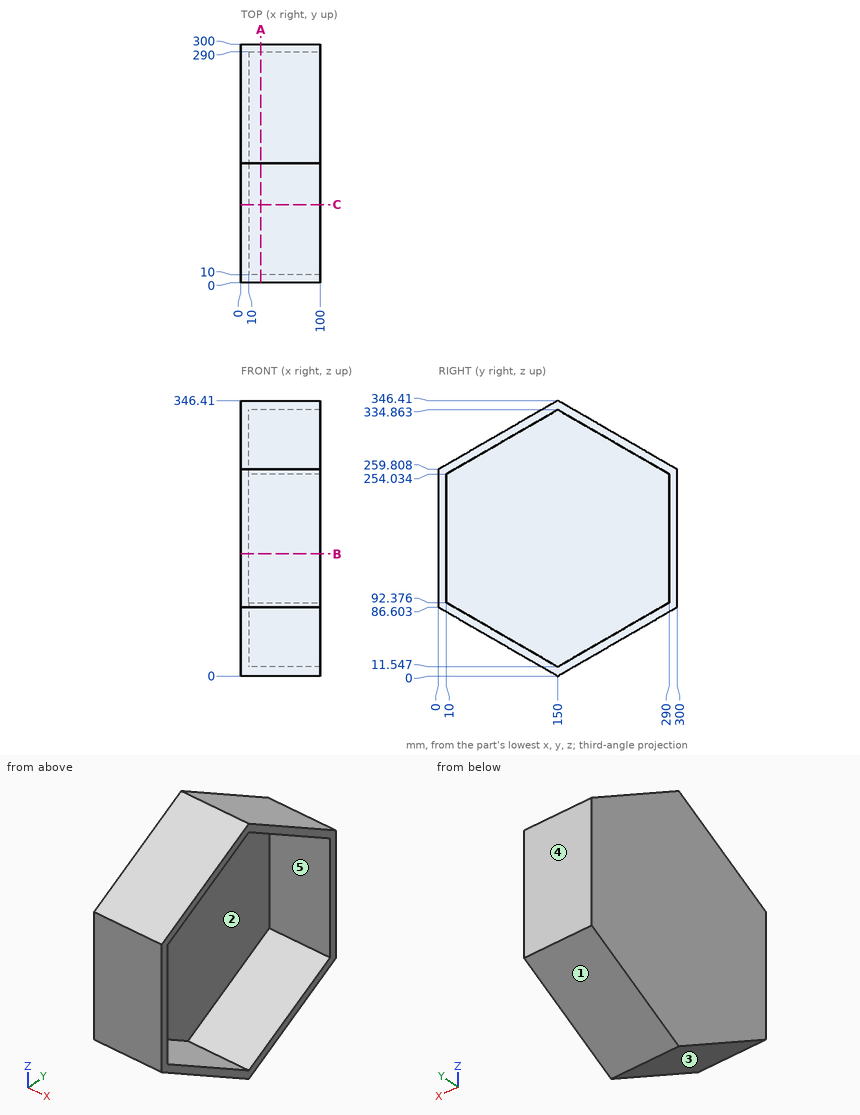
Here's the drawing with two shaded views (mm, measured from the low corner). I have some questions. A direction names the side the tool comes from. Coordinates: 2 decimals unless noted, no trailing zeros. Loops run counter-clockwise (first coordinate to the right, second up) from the corner with the lowest first, then second, coordinate; pieces in that order, holes last. Notation, with made-up numbers: M 85.5,37.5 L 98.5,37.5 A21 ccw 98.5,73.5 Z; hole C 88,28 d10. An arc over 180 degrees is marked long. Put each result on its own line as item: value. Start each with the question number.
(1) We'd pull the mould along Y, two halves only. Please class the marked faces 3, 4 and 5: +Y half, -Y half, draft (parallel to the pull), parting line (faces both ways), or undercut.
(2) Which directions (+Z, -Z, +X, -X, +Y, -Y) give clear straight access to the entire face, cutting with the end or side of a thin tool? Please do the marked faces 1 and 2.
(3) Will these pins go through, and if not, where does the flat tip stop? pin 1 Ø8 at (x, y) = (16.5, 69.5) entering from -Z; pin 2 Ø1.5 at (x, y) = (64.5, 212) entering from -Z; pin 3 Ø6 at (y, z) = (123.5, 150) entering from +X.
(4) I need wall thicknesses on probe 1 along Y at (x, z) = (16, 205); probe 2 along Z at (x, y) = (51.5, 152) (1 decimal); probe 3 along X at (y, z) = (135, 302). Which ranges of each line are inside material? Lowest first, please.
(5) Imagine slicing it at A-A on x = 25. List the corners of the cut face in (y, z) for me (1 decimal), and give its area (3 significant figures).
(6) Imagine slicing it at C-C on y = 98. List the corners of the cut face in (x, z) for me, and give its area (3 significant figures).
(7) Imagine slicing it at B-B on z = 153.5. List the corners of the cut face in (x, y) for me.
Worked answers:
1. face 3: -Y half
1. face 4: +Y half
1. face 5: undercut
2. face 1: -Z, +X, -X, +Y
2. face 2: +X
3. pin 1: stops at z = 44.17
3. pin 2: stops at z = 35.36
3. pin 3: stops at x = 10
4. probe 1: y = 0 to 10, 290 to 300
4. probe 2: z = 1.2 to 12.7, 333.7 to 345.3
4. probe 3: x = 0 to 10
5. outline: M 0,86.6 L 150,0 L 300,86.6 L 300,259.8 L 150,346.4 L 0,259.8 Z; hole M 10,92.4 L 150,11.5 L 290,92.4 L 290,254 L 150,334.9 L 10,254 Z
5. area: 10,000 mm2
6. outline: M 0,30.02 L 100,30.02 L 100,41.57 L 10,41.57 L 10,304.84 L 100,304.84 L 100,316.39 L 0,316.39 Z
6. area: 4,940 mm2
7. outline: M 0,0 L 100,0 L 100,10 L 10,10 L 10,290 L 100,290 L 100,300 L 0,300 Z
